Model file for the job. Use its own axes, mm. Coordinates: 2 decimals unless noted, no trailing zeros. Write each loop counter-clockwise with the first axis right and the second up, starting at its lowest first coordinate (ties: lowest second). Pieces come first, ordered by that corner, then holes. Notation, with made-up numbers: (-17.5, -26) - (13.5, -26) arc R11 cw to (13.5, -22) - close; hole circle Ø3 at (-14, -39). An arc over 180 degrees is marked (long way). Put each result on its own line as item: value. Start each with the question number.
1. Drop flat-ended pins along their axis: P1, Ø1.6, axis at y = 39.5, z = 2, coming from the -X side; P2, Ø1.6, axis at x = -26.5, z = 3, coming from the +Y side; P3, Ø10, axis at x = -63.5, y = -17, coming from the -Z side; P4, Ø2, axis at x = -48.5, z = 4.5, coming from the +Y side. Give the stop position or say it passes through.
2. Saw through at A-A, the plane x = -32. Write the cut outline in (y, z).
3. Saw through at C-C, the plane z = 2.25. Give the number of separate pieces and of enclosed holes in the cut face, plus the area to 3 significant figures.
4. Saw through at D-D, the plane y = 11.5. Write the cut outline in (x, z), plus the area to 3 significant figures.
5. Saw through at B-B, the plane y = -62.5. Write the cut outline in (x, z).
6. Drill centre lines: L1, parallel to Y at x = -42, z = 0.35; L2, parallel to Y at x = 8.5, z = 2.15; L3, parallel to Y at x = -36.5, z = 1.2. Where is each one in solid material? Low to high. Write a range as from..to.
```python
from build123d import *

# Parameters (mm, degrees)
SKETCH1_W           = 52.07
SKETCH1_H           = 112.776
BOSS_EXTRUDE1_DEPTH = 5.334
SKETCH2_W           = 5.334
SKETCH2_H           = 16.110857143
SKETCH2_H_2         = 16.110857142
CUT_EXTRUDE1_DEPTH  = 82.040197417
CUT_EXTRUDE2_DEPTH  = 82.040197417
SKETCH5_W           = 5.334
SKETCH5_H           = 16.110857143
BOSS_EXTRUDE2_DEPTH = 38.1
SKETCH6_W           = 12.7
SKETCH6_H           = 5.334
BOSS_EXTRUDE3_DEPTH = 5.334
SKETCH7_W           = 20.804949133
SKETCH7_H           = 5.334
CUT_EXTRUDE4_DEPTH  = 106.172156174
SKETCH8_W           = 5.334
SKETCH8_H           = 6.622142857
BOSS_EXTRUDE4_DEPTH = 11.43
SKETCH9_W           = 20.828
SKETCH9_H           = 5.334
CUT_EXTRUDE5_DEPTH  = 106.172156174
SKETCH10_W          = 5.334
SKETCH10_H          = 4.154714286
BOSS_EXTRUDE5_DEPTH = 11.684


with BuildPart() as part:
    # Sketch1 → Boss-Extrude1 (new body)
    with BuildSketch(Plane.XY):
        with Locations((-13.887031982, -13.934780119)):
            Rectangle(SKETCH1_W, SKETCH1_H)
    extrude(amount=BOSS_EXTRUDE1_DEPTH)

    # Sketch2 → Cut-Extrude1 (cut, through all)
    with BuildSketch(Plane.XY.offset(5.334)):
        with Locations((-37.255031982, 18.286934167)):
            Rectangle(SKETCH2_W, SKETCH2_H)
        with Locations((-37.255031982, -13.93478012)):
            Rectangle(SKETCH2_W, SKETCH2_H)
        with Locations((-37.255031982, -46.156494405)):
            Rectangle(SKETCH2_W, SKETCH2_H_2)
        with Locations((9.480968018, -46.156494405)):
            Rectangle(SKETCH2_W, SKETCH2_H_2)
        with Locations((9.480968018, -13.93478012)):
            Rectangle(SKETCH2_W, SKETCH2_H)
        with Locations((9.480968018, 18.286934167)):
            Rectangle(SKETCH2_W, SKETCH2_H)
    extrude(amount=-CUT_EXTRUDE1_DEPTH, mode=Mode.SUBTRACT)

    # Sketch3 → Cut-Extrude2 (cut, through all)
    with BuildSketch(Plane.XY.offset(5.334)):
        Polygon((-22.544809753, -41.442678073), (-13.491049115, -50.348823048), (-17.231630005, -54.151402516), (-26.285390642, -45.245257541), align=None)
        Polygon((-22.544809753, -51.602678073), (-13.491049115, -60.508823048), (-17.231630005, -64.311402516), (-26.285390642, -55.405257541), align=None)
        Polygon((-12.384809753, -51.602678073), (-3.331049115, -60.508823048), (-7.071630005, -64.311402516), (-16.125390642, -55.405257541), align=None)
    extrude(amount=-CUT_EXTRUDE2_DEPTH, mode=Mode.SUBTRACT)

    # Sketch5 → Boss-Extrude2 (add)
    with BuildSketch(Plane.ZY.offset(39.922031982)):
        with Locations((2.667, -30.045637263)):
            Rectangle(SKETCH5_W, SKETCH5_H)
    extrude(amount=BOSS_EXTRUDE2_DEPTH)

    # Sketch6 → Boss-Extrude3 (add)
    with BuildSketch(Plane(origin=(0, -21.990208691, 0), x_dir=(1, 0, 0), z_dir=(0, 1, 0))):
        with Locations((-58.972031982, -2.667)):
            Rectangle(SKETCH6_W, SKETCH6_H)
    extrude(amount=BOSS_EXTRUDE3_DEPTH)

    # Sketch7 → Cut-Extrude4 (cut, through all)
    with BuildSketch(Plane.XY.offset(5.334)):
        with Locations((-29.519557416, 3.409791309)):
            Rectangle(SKETCH7_W, SKETCH7_H)
    extrude(amount=-CUT_EXTRUDE4_DEPTH, mode=Mode.SUBTRACT)

    # Sketch8 → Boss-Extrude4 (add)
    with BuildSketch(Plane.ZY.offset(39.922031982)):
        with Locations((2.667, -2.56828012)):
            Rectangle(SKETCH8_W, SKETCH8_H)
    extrude(amount=BOSS_EXTRUDE4_DEPTH)

    # Sketch9 → Cut-Extrude5 (cut, through all)
    with BuildSketch(Plane.XY.offset(5.334)):
        with Locations((-29.508031982, 39.786219881)):
            Rectangle(SKETCH9_W, SKETCH9_H)
    extrude(amount=-CUT_EXTRUDE5_DEPTH, mode=Mode.SUBTRACT)

    # Sketch10 → Boss-Extrude5 (add)
    with BuildSketch(Plane.ZY.offset(39.922031982)):
        with Locations((2.667, 8.154148452)):
            Rectangle(SKETCH10_W, SKETCH10_H)
    extrude(amount=BOSS_EXTRUDE5_DEPTH)


solid = part.part
```
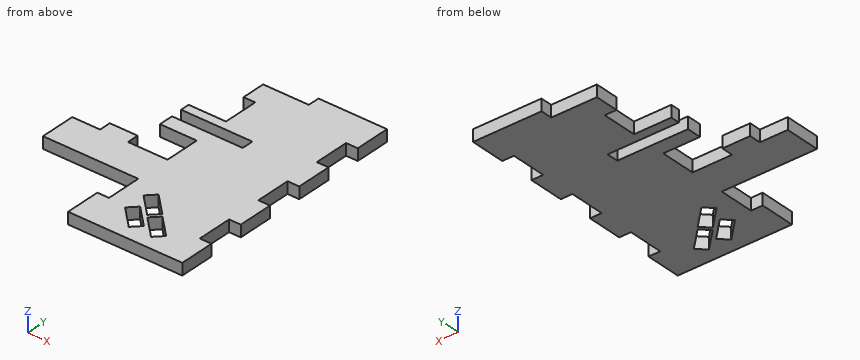
Final values:
1. P1: stops at x = -19.09
1. P2: stops at y = 37.12
1. P3: stops at z = 0
1. P4: stops at y = 10.23
2. outline: (-70.32, 0) - (0.74, 0) - (0.74, 5.33) - (-70.32, 5.33) - close; (6.08, 0) - (37.12, 0) - (37.12, 5.33) - (6.08, 5.33) - close
3. separate pieces: 1
3. enclosed holes: 3
3. area: 5,740 mm²
4. outline: (-34.59, 0) - (6.81, 0) - (6.81, 5.33) - (-34.59, 5.33) - close
4. area: 221 mm²
5. outline: (-39.92, 0) - (-19.07, 0) - (-19.07, 5.33) - (-39.92, 5.33) - close; (-15.45, 0) - (-8.91, 0) - (-8.91, 5.33) - (-15.45, 5.33) - close; (-5.29, 0) - (12.15, 0) - (12.15, 5.33) - (-5.29, 5.33) - close
6. L1: y = -38.1..-21.99, -5.88..0.74, 6.08..10.23
6. L2: y = -70.32..-54.21, -38.1..-21.99, -5.88..10.23, 26.34..42.45
6. L3: y = -70.32..-54.21, -38.1..-21.99, -5.88..0.74, 6.08..10.23, 26.34..37.12
